```python
from build123d import *

# Parameters (mm, degrees)
F0_R     = 26
F1_DEPTH = 4
F2_R     = 25
F3_DEPTH = 2
F4_R     = 0.99999
F5_R     = 0.5
F6_W     = 4
F6_H     = 45
F7_DEPTH = 2


# Not quite as in the source:
# - a fillet or chamfer is up to 0.001 mm smaller than in the source, because OpenCascade refuses the exact size


with BuildPart() as f1:
    # F0 (on Front) → F1 (new body)
    with BuildSketch(Plane.XZ):
        Circle(F0_R)
    extrude(amount=F1_DEPTH)

    # F2 (on face) → F3 (join)
    with BuildSketch(Plane(origin=(0, 0, 0), x_dir=(-1, 0, 0), z_dir=(0, 1, 0))):
        Circle(F2_R)
    extrude(amount=F3_DEPTH)

    # F4 (radius 1 in the source; OpenCascade refuses exactly that, so slightly less here)
    f4_edges = [f1.edges().sort_by_distance(p)[0] for p in [
        (-26, 0, 0),
    ]]
    fillet(f4_edges, radius=F4_R)

    # F5
    f5_edges = [f1.edges().sort_by_distance(p)[0] for p in [
        (25, 2, 0),
    ]]
    fillet(f5_edges, radius=F5_R)

    # F6 (on face) → F7 (cut)
    with BuildSketch(Plane(origin=(0, 2, 0), x_dir=(-1, 0, 0), z_dir=(0, 1, 0))):
        Rectangle(F6_W, F6_H)
    extrude(amount=-F7_DEPTH, mode=Mode.SUBTRACT)


solid = f1.part
```
Input: part model. Units: mm. Frame: model coordinates. A direction names the side the tool comes from. Round coordinates to 2 decimals unless told otherwise and drop trailing zeros. Order: outer loops, then holes, each group sorted by start corner. A loop starts at its lowest first (then second) coordinate and runs counter-clockwise, first axis right, second up. Notation, with made-up numbers: (31.25, 86) - (71.25, 86) arc R19 cw to (71.25, 103) - close; hole circle Ø6 at (14.5, -15.5). An arc over 180 degrees is marked (long way). Answer in a Markdown table with one row per item.
Item 1: Pin query (flat end, axial travel): pin 1 (1 mm diameter, centred on y = 1, z = 7.5, fed in from -X); pin 2 (3 mm diameter, centred on y = -2, z = -18.5, fed in from +X); pin 3 (1 mm diameter, centred on x = 5, y = -1.5, fed in from +Z). Return the tip coordinate at first contact, or that it passes through.
Model answer:
| item | result |
|---|---|
| pin 1 | stops at x = -24 |
| pin 2 | stops at x = 19.67 |
| pin 3 | stops at z = 25.61 |
Item 2: Section query C-C (y = -2.6). Return the cut outline in (x, z).
Model answer:
| item | result |
|---|---|
| outline | circle Ø52 at (0, 0) |
Item 3: Mould query, pull axis X, two halves, no side actions, for faces 1 (the flat face through (0, -4, 0)), 2 (the cylindrical face through (-20.633, -2.479, -15.821)), 3 (the flat face through (0, 0, 0)). Classes: released by +X, released by -X, zero draft, split by the parting line, or undercut.
Model answer:
| item | result |
|---|---|
| face 1 | zero draft |
| face 2 | split by the parting line |
| face 3 | undercut |
Item 4: Reachability of faces 4 (the flat face through (2, 1, 0)), 5 (the flat face through (-5, 2, 0)) from +Z, -Z, +X, -X, +Y, -Y: full face, straight path, thin tool, end or side. Return the list, or none.
Model answer:
| item | result |
|---|---|
| face 4 | +Y |
| face 5 | +Z, -Z, +X, -X, +Y |
Item 5: Line query: line 1 (Z direction, x = 0, y = 1.3); line 2 (X direction, y = 0.7, z = -16.5); line 3 (X direction, y = 0.85, z = 5.5). Output: solid intervals per line, ascending.
Model answer:
| item | result |
|---|---|
| line 1 | z = -25 to -22.5, 22.5 to 25 |
| line 2 | x = -18.78 to -2, 2 to 18.78 |
| line 3 | x = -24.39 to -2, 2 to 24.39 |
